Design review of the part built by this model. Coordinates are the model's own, in mm. Face numbers are marked on the shaded views. A direction names the side the tool comes from. Give positions to 0.01 mm unless a question says otherwise; leave off trailing zeros. Loops run counter-clockwise (first coordinate to the right, second up) from the corner with the lowest first, then second, coordinate; pieces in that order, holes last. Notation, with made-up numbers: (15.25, 86.5) -> (70.25, 86.5) arc R21 ccw to (70.25, 102.5) -> close; hole circle Ø7 at (19, -36.75). An arc over 180 degrees is marked (long way). Use a Markdown table: item, result. Add a question column.
1. Add section B-B (y = -172). State the section outline as (x, z) points.
2. Add section C-C (y = -44). State the section outline as (x, z) points, and give its area (3 significant figures).
3. For pin 1 Ø4 at (x, y) = (-2.5, -131) entering from +Z; pin 2 Ø6 at (y, z) = (-20, 0) entering from -X; pin 3 Ø2 at (y, z) = (-175.5, 8.5) entering from +X; pin 4 Ø7.5 at (y, z) = (-172, 0) entering from +X, all flat-tipped, find the tip position at first contact; note any pin that passes through.
4. For the marked faces 1 and 2, list the 3-axis set-ups (+Z, -Z, +X, -X, +Y, -Y) from which the entire face can be reached by the end or side of a thin tool; tool diameter is ignored.
5. To check wall thickness, follow line 1 (Y direction, x = -4.25, z = 0); line 2 (Y direction, x = -9.25, z = 0); line 3 (Z direction, x = 0.25, y = -205). State the ranges of each line that lie inside material, in increasing order.
6. Add section A-A (y = -20). State the section outline as (x, z) points.
7. Add section D-D (z = 0). Count the separate pieces of the cut face and the enclosed holes in it, and give its area (3 significant figures).
```python
from build123d import *

# Parameters (mm, degrees)
EXTRUDE_1_DEPTH              = 195
EXTRUDE_2_DEPTH              = 20
CUT_EXTRUDE_5_DEPTH          = 20
CUT_EXTRUDE_5_DEPTH_BACK     = 20
HOLE_WIZARD_M6_1_D           = 5
HOLE_WIZARD_M6_1_CSINK_D     = 6.05
HOLE_WIZARD_M6_1_CSINK_ANGLE = 90
HOLE_WIZARD_1_D              = 6.5
HOLE_WIZARD_1_CBORE_D        = 12
HOLE_WIZARD_1_CBORE_DEPTH    = 15
HOLE_WIZARD_2_D              = 6.5
HOLE_WIZARD_2_CBORE_D        = 12
HOLE_WIZARD_2_CBORE_DEPTH    = 12


with BuildPart() as part:
    # Sketch 1 → Extrude 1 (new body)
    with BuildSketch(Plane(origin=(0, 0, 0), x_dir=(1, 0, 0), z_dir=(0, 1, 0))):
        Polygon((0, 13.856406461), (-12, 6.92820323), (-12, -6.92820323), (0, -13.856406461), (12, -6.92820323), (12, 6.92820323), align=None)
    extrude(amount=-EXTRUDE_1_DEPTH)

    # Sketch 3 → Extrude 2 (add)
    with BuildSketch(Plane.XZ.offset(195)):
        with BuildLine():
            Line((6.7, 3.620773398), (6.7, -3.620773398))
            ThreePointArc((6.7, -3.620773398), (5.920485754, -6.301724722), (3.825, -8.146740146))
            ThreePointArc((3.825, -8.146740146), (-9, 0), (3.825, 8.146740146))
            ThreePointArc((3.825, 8.146740146), (5.920485754, 6.301724722), (6.7, 3.620773398))
        make_face()
    extrude(amount=EXTRUDE_2_DEPTH)

    # Sketch 5 → Cut-Extrude 5 (cut, two sides: drawn at the far end of the back side and taken through both)
    with BuildSketch(Plane.XY.offset(-CUT_EXTRUDE_5_DEPTH_BACK)):
        with BuildLine():
            ThreePointArc((12, -3.560911085), (0, 0), (-12, -3.560911085))
            Line((-12, -3.560911085), (-17.888682829, 19.552850293))
            Line((-17.888682829, 19.552850293), (25.347523703, 18.415156831))
            Line((25.347523703, 18.415156831), (12, -3.560911085))
        make_face()
    extrude(amount=CUT_EXTRUDE_5_DEPTH + CUT_EXTRUDE_5_DEPTH_BACK, mode=Mode.SUBTRACT)

    # Hole Wizard M6 _1 (through all)
    with Locations(Plane(origin=(6.7, 0, 0), x_dir=(0, 0, -1), z_dir=(1, 0, 0))):
        with Locations((0, -205)):
            CounterSinkHole(HOLE_WIZARD_M6_1_D / 2, HOLE_WIZARD_M6_1_CSINK_D / 2, counter_sink_angle=HOLE_WIZARD_M6_1_CSINK_ANGLE)

    # Hole Wizard 1 (through all)
    with Locations(Plane(origin=(12, 0, 0), x_dir=(0, 0, -1), z_dir=(1, 0, 0))):
        with Locations((0, -172)):
            CounterBoreHole(HOLE_WIZARD_1_D / 2, HOLE_WIZARD_1_CBORE_D / 2, HOLE_WIZARD_1_CBORE_DEPTH)

    # Hole Wizard 2 (through all)
    with Locations(Plane(origin=(12, 0, 0), x_dir=(0, 0, -1), z_dir=(1, 0, 0))):
        with Locations((0, -75), (0, -20)):
            CounterBoreHole(HOLE_WIZARD_2_D / 2, HOLE_WIZARD_2_CBORE_D / 2, HOLE_WIZARD_2_CBORE_DEPTH)


solid = part.part
```
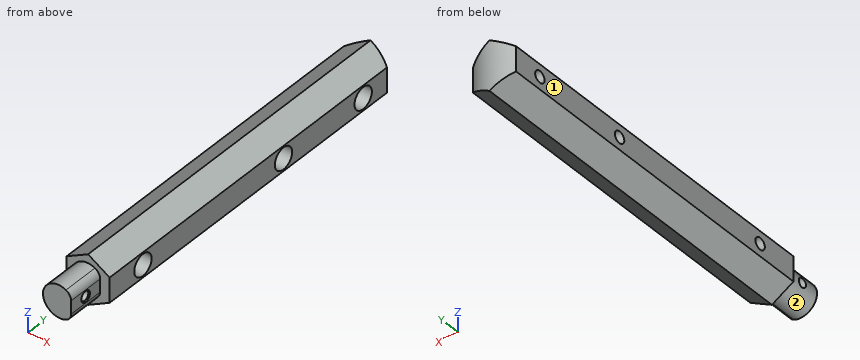
Taken from the geometry:
| question | item | result |
|---|---|---|
| 1 | outline | (-12, -6.93) -> (0, -13.86) -> (12, -6.93) -> (12, -6) -> (-3, -6) -> (-3, -3.25) -> (-12, -3.25) -> close; (-12, 3.25) -> (-3, 3.25) -> (-3, 6) -> (12, 6) -> (12, 6.93) -> (0, 13.86) -> (-12, 6.93) -> close |
| 2 | outline | (-12, -6.93) -> (0, -13.86) -> (12, -6.93) -> (12, 6.93) -> (0, 13.86) -> (-12, 6.93) -> close |
| 2 | area | 499 mm^2 |
| 3 | pin 1 | stops at z = 13.57 |
| 3 | pin 2 | passes through |
| 3 | pin 3 | stops at x = 11.01 |
| 3 | pin 4 | stops at x = -3 |
| 4 | face 1 | +Z, -Z, -X, +Y, -Y |
| 4 | face 2 | -Y |
| 5 | line 1 | y = -215 to -207.5, -202.5 to -175.25, -168.75 to -78.25, -71.75 to -23.25, -16.75 to -0.41 |
| 5 | line 2 | y = -195 to -175.25, -168.75 to -78.25, -71.75 to -23.25, -16.75 to -2.04 |
| 5 | line 3 | z = -9 to -2.5, 2.5 to 9 |
| 6 | outline | (-12, -6.93) -> (0, -13.86) -> (12, -6.93) -> (12, -6) -> (0, -6) -> (0, -3.25) -> (-12, -3.25) -> close; (-12, 3.25) -> (0, 3.25) -> (0, 6) -> (12, 6) -> (12, 6.93) -> (0, 13.86) -> (-12, 6.93) -> close |
| 7 | separate pieces | 5 |
| 7 | enclosed holes | 0 |
| 7 | area | 4,210 mm^2 |
